Model file for the job. Use its own axes, mm. A direction names the side the tool comes from. Give positions to 0.01 mm unless a question says otherwise; leave off trailing zeros. Order: outer loops, then holes, each group sorted by start corner. A loop starts at its lowest first (then second) coordinate and runs counter-clockwise, first axis right, second up. Notation, with made-up numbers: (50, -0.75) -> (96, -0.75) arc R8 cw to (96, 9.25) -> close; hole circle Ø1 at (11, 27.25). An arc over 180 degrees is marked (long way). Answer in a Markdown table with one row per item. Add a question column.
from build123d import *

# Parameters (mm, degrees)
SKETCH1_W                      = 35
SKETCH1_H                      = 35
BOSS_EXTRUDE1_DEPTH            = 20
CUT_EXTRUDE1_DEPTH             = 21
M4X0_7_TAPPED_HOLE1_AT_2_COUNT = 2
M4X0_7_TAPPED_HOLE1_AT_2_PITCH = 22.360679775
M4X0_7_TAPPED_HOLE1_AT_3_COUNT = 2
M4X0_7_TAPPED_HOLE1_AT_3_PITCH = 20
M4X0_7_TAPPED_HOLE1_AT_4_COUNT = 2
M4X0_7_TAPPED_HOLE1_AT_4_PITCH = 10


with BuildPart() as part:
    # Sketch1 → Boss-Extrude1 (new body)
    with BuildSketch(Plane.XY):
        with Locations((-17.5, 17.5)):
            Rectangle(SKETCH1_W, SKETCH1_H)
    extrude(amount=BOSS_EXTRUDE1_DEPTH)

    # Sketch2 → Cut-Extrude1 (cut, through all)
    with BuildSketch(Plane.XY.offset(20)):
        with BuildLine():
            ThreePointArc((-15.9125, 23.648361062), (-17.5, 23.85), (-19.0875, 23.648361062))
            Line((-19.0875, 23.648361062), (-19.0875, 22.2625))
            Line((-19.0875, 22.2625), (-15.9125, 22.2625))
            Line((-15.9125, 22.2625), (-15.9125, 23.648361062))
        make_face()
        with BuildLine():
            Line((-19.0875, 22.2625), (-19.0875, 23.648361062))
            ThreePointArc((-19.0875, 23.648361062), (-21.388564967, 12.479884214), (-11.15, 17.5))
            ThreePointArc((-11.15, 17.5), (-12.479884214, 21.388564967), (-15.9125, 23.648361062))
            Line((-15.9125, 23.648361062), (-15.9125, 22.2625))
            Line((-15.9125, 22.2625), (-19.0875, 22.2625))
        make_face()
        with BuildLine():
            Line((-15.9125, 25.4375), (-19.0875, 25.4375))
            Line((-19.0875, 25.4375), (-19.0875, 23.648361062))
            ThreePointArc((-19.0875, 23.648361062), (-17.5, 23.85), (-15.9125, 23.648361062))
            Line((-15.9125, 23.648361062), (-15.9125, 25.4375))
        make_face()
    extrude(amount=-CUT_EXTRUDE1_DEPTH, mode=Mode.SUBTRACT)

    # Sketch4 → M4x0.7 Tapped Hole1 (revolve, cut)
    with BuildSketch(Plane(origin=(-35, 27.5, 5), x_dir=(0, 0, 1), z_dir=(0, 1, 0))):
        Polygon((0, 0), (0, 10.991420021), (1.65, 10), (1.65, 0), align=None)
    m4x0_7_tapped_hole1 = revolve(axis=Axis((-41.35, 27.5, 5), (1, 0, 0)), mode=Mode.SUBTRACT)

    # M4x0.7 Tapped Hole1 at 2: M4x0.7 Tapped Hole1 ×2
    with Locations(*[Vector(0, -0.894427191, 0.447213595) * (i * M4X0_7_TAPPED_HOLE1_AT_2_PITCH) for i in range(1, M4X0_7_TAPPED_HOLE1_AT_2_COUNT)]):
        add(m4x0_7_tapped_hole1, mode=Mode.SUBTRACT)

    # M4x0.7 Tapped Hole1 at 3: M4x0.7 Tapped Hole1 ×2
    with Locations(*[(0, -i * M4X0_7_TAPPED_HOLE1_AT_3_PITCH, 0) for i in range(1, M4X0_7_TAPPED_HOLE1_AT_3_COUNT)]):
        add(m4x0_7_tapped_hole1, mode=Mode.SUBTRACT)

    # M4x0.7 Tapped Hole1 at 4: M4x0.7 Tapped Hole1 ×2
    with Locations(*[(0, 0, i * M4X0_7_TAPPED_HOLE1_AT_4_PITCH) for i in range(1, M4X0_7_TAPPED_HOLE1_AT_4_COUNT)]):
        add(m4x0_7_tapped_hole1, mode=Mode.SUBTRACT)

    # Mirror1: M4x0.7 Tapped Hole1 across plane
    add(m4x0_7_tapped_hole1.mirror(Plane.ZY.offset(17.5)), mode=Mode.SUBTRACT)

    # Mirror1 copy 1 sketch → Mirror1 copy 1 (revolve, cut)
    with BuildSketch(Plane(origin=(0, 7.5, 15), x_dir=(0, 0, 1), z_dir=(0, 1, 0))):
        Polygon((0, 0), (0, -10.991420021), (1.65, -10), (1.65, 0), align=None)
    revolve(axis=Axis((6.35, 7.5, 15), (1, 0, 0)), mode=Mode.SUBTRACT)

    # Mirror1 copy 2 sketch → Mirror1 copy 2 (revolve, cut)
    with BuildSketch(Plane(origin=(0, 7.5, 5), x_dir=(0, 0, 1), z_dir=(0, 1, 0))):
        Polygon((0, 0), (0, -10.991420021), (1.65, -10), (1.65, 0), align=None)
    revolve(axis=Axis((6.35, 7.5, 5), (1, 0, 0)), mode=Mode.SUBTRACT)

    # Mirror1 copy 3 sketch → Mirror1 copy 3 (revolve, cut)
    with BuildSketch(Plane(origin=(0, 27.5, 15), x_dir=(0, 0, 1), z_dir=(0, 1, 0))):
        Polygon((0, 0), (0, -10.991420021), (1.65, -10), (1.65, 0), align=None)
    revolve(axis=Axis((6.35, 27.5, 15), (1, 0, 0)), mode=Mode.SUBTRACT)


solid = part.part
Item 1: Saw through at B-B on z = 12.5. List the corners of the cut face in (x, y).
Item 2: Wall check: line 1 (Z direction, x = -28, y = 7.5); line 2 (Y direction, x = -27.5, z = 5); line 3 (X direction, y = 25, z = 16). Give the ranges that are in metal, low to high.
Item 3: Saw through at A-A on x = -17.5. List the corners of the cut face in (y, z).
Item 4: Two-plate mould, pull along Y, no slides. Class faces 1 (the flat face through (-35, 17, 10)), 2 (the conical face through (-24.2, 27.4, 15.3)), 3 (the flat face through (-18, 0, 10)): pulls with the +Y half, pulls with the -Y half, needs draft (parallel to the pull), parting line crosses it, or undercut.
Item 5: Pin check, flat tips, straight feed: pin 1 Ø2.5 at (y, z) = (27.5, 15) entering from +X; pin 2 Ø2 at (y, z) = (27.5, 5) entering from -X; pin 3 Ø3 at (y, z) = (7.5, 15) entering from +X. Stop position of each tip, or through.
Item 6: Which spindle directions (+Z, -Z, +X, -X, +Y, -Y) get a long thin tool onto all of the face, cutting with end or side? Do faces 4 (the flat face through (-15.912, 25, 10)), 5 (the cylindrical face through (-30.07, 25.864, 4.785)), 6 (the cylindrical face through (-4.93, 8.132, 16.524)). Say none if no direction does.
Evaluation:
| question | item | result |
|---|---|---|
| 1 | outline | (-35, 0) -> (0, 0) -> (0, 35) -> (-35, 35) -> close; hole (-19.09, 23.65) arc R6.35 ccw (long way) to (-15.91, 23.65) -> (-15.91, 25.44) -> (-19.09, 25.44) -> close |
| 2 | line 1 | z = 0 to 3.35, 6.65 to 13.35, 16.65 to 20 |
| 2 | line 2 | y = 0 to 5.85, 9.15 to 25.85, 29.15 to 35 |
| 2 | line 3 | x = -35 to -19.09, -15.91 to 0 |
| 3 | outline | (0, 0) -> (11.15, 0) -> (11.15, 20) -> (0, 20) -> close; (25.44, 0) -> (35, 0) -> (35, 20) -> (25.44, 20) -> close |
| 4 | face 1 | needs draft |
| 4 | face 2 | undercut |
| 4 | face 3 | pulls with the -Y half |
| 5 | pin 1 | stops at x = -10.24 |
| 5 | pin 2 | stops at x = -24.61 |
| 5 | pin 3 | stops at x = -10.09 |
| 6 | face 4 | +Z, -Z |
| 6 | face 5 | -X |
| 6 | face 6 | +X |
